Answer from the drawing. Dimensions are ordinates in mm from the lowest x, y and z of the part. A direction names the side the tool comes from. Give positions to 0.01 mm unless a question says otherwise; leave off trailing zeros. Loops run counter-clockwise (first coordinate to the right, second up) from the corner with the lowest first, then second, coordinate; pieces in that order, holes last. Notation, with made-up numbers: (84, -26.5) -> (108, -26.5) arc R23 cw to (108, 2.5) -> close; hole circle Ø6 at (10, 76.5). An arc over 180 degrees is marked (long way). Write each question's results on one line, items separated by ' | '. Start each with the question number.
Item 1: Section A-A on x = 18 is taken. Write down the section's boundary in (y, z).
Item 2: Each of these flat-tipped pins is pushed along its axis until it touches: P1, Ø1, axis at x = 13.5, y = 19.5, coming from the +Z side; P2, Ø4.5, axis at x = 21, z = 21, coming from the +Y side. Where does it stop, or does it pass through?
Item 3: Section B-B on y = 65 is taken. Write down the section's boundary in (x, z), and give its area (3 significant figures).
Item 4: Determine the mould class of the marked faces 1, 2 and 3 for opening direction Y: +Y half, -Y half, draft (parallel to the pull), parting line (faces both ways), or undercut.
Item 5: Which of the six approach directions +Z, -Z, +X, -X, +Y, -Y give full straight-line access (tool end or side, diameter ignored) to the marked faces 4 and 5?
Item 6: Find the intervals of material crossed by line 1 (X direction, y = 2.5, z = 15); line 2 (Y direction, x = 37, z = 1.95); line 3 (Z direction, x = 6, y = 2), in increasing order.
Item 7: Section D-D on z = 3.5 is taken. Write down the section's boundary in (x, y).
Item 8: Section C-C on x = 6 is taken. Write down the section's boundary in (y, z), and give its area (3 significant figures).
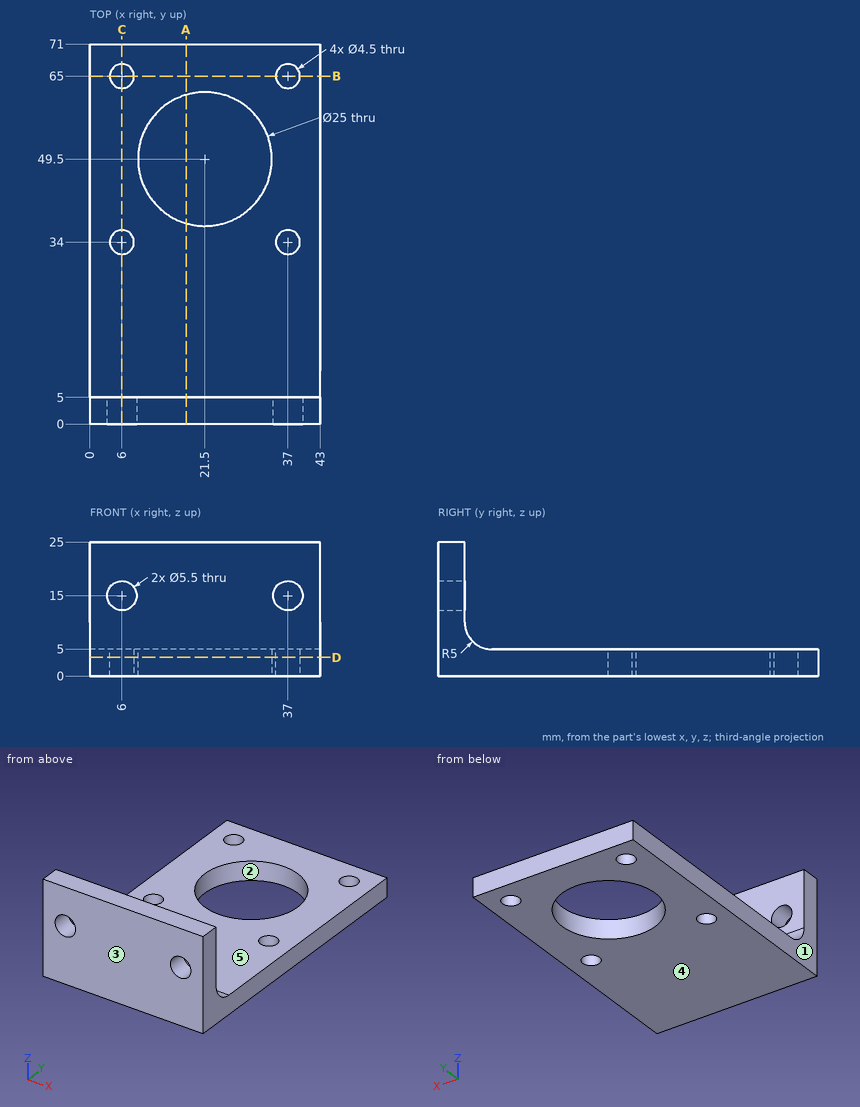
Findings:
1) outline: (0, 0) -> (37.5, 0) -> (37.5, 5) -> (10, 5) arc R5 cw to (5, 10) -> (5, 25) -> (0, 25) -> close; (61.5, 0) -> (71, 0) -> (71, 5) -> (61.5, 5) -> close
2) P1: z = 5 | P2: y = 5
3) outline: (0, 0) -> (3.75, 0) -> (3.75, 5) -> (0, 5) -> close; (8.25, 0) -> (34.75, 0) -> (34.75, 5) -> (8.25, 5) -> close; (39.25, 0) -> (43, 0) -> (43, 5) -> (39.25, 5) -> close | area: 170 mm2
4) face 1: draft | face 2: undercut | face 3: -Y half
5) face 4: -Z, +X, -X, +Y, -Y | face 5: +Z, +X, -X, +Y
6) line 1: 0 to 3.25, 8.75 to 34.25, 39.75 to 43 | line 2: 0 to 31.75, 36.25 to 62.75, 67.25 to 71 | line 3: 0 to 12.25, 17.75 to 25
7) outline: (0, 0) -> (43, 0) -> (43, 71) -> (0, 71) -> close; hole circle Ø4.5 at (6, 34); hole circle Ø4.5 at (6, 65); hole circle Ø25 at (21.5, 49.5); hole circle Ø4.5 at (37, 34); hole circle Ø4.5 at (37, 65)
8) outline: (0, 0) -> (31.75, 0) -> (31.75, 5) -> (10, 5) arc R5 cw to (5, 10) -> (5, 12.25) -> (0, 12.25) -> close; (0, 17.75) -> (5, 17.75) -> (5, 25) -> (0, 25) -> close; (36.25, 0) -> (62.75, 0) -> (62.75, 5) -> (36.25, 5) -> close; (67.25, 0) -> (71, 0) -> (71, 5) -> (67.25, 5) -> close | area: 388 mm2
